CAD build for the part. Positions are in the model's coordinates, mm. Face numbers are marked on the shaded views. A direction names the side the tool comes from. Round coordinates to 2 decimals unless told otherwise and drop trailing zeros. Order: outer loops, then holes, each group sorted by start corner. A loop starts at its lowest first (then second) coordinate and runs counter-clockwise, first axis right, second up. Notation, with made-up numbers: (50, 20) -> (64, 20) arc R22 cw to (64, 26) -> close; hole circle Ø8 at (-12.5, -38). An arc over 180 degrees is marked (long way). Answer as CSV lines item,"result". Start each with the question number.
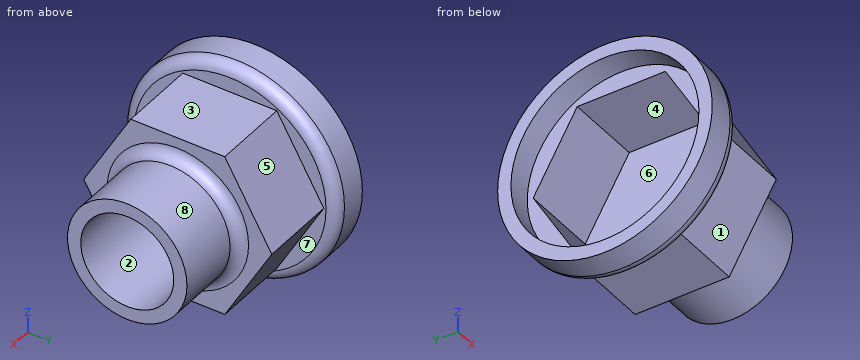
from build123d import *

# Parameters (mm, degrees)
F3_DEPTH = 7
F4_R     = 10.135693
F5_DEPTH = 13.801
F6_R     = 1
F7_R     = 1
F8_R     = 4.2
F9_DEPTH = 0.2


with BuildPart() as f1:
    # F0 (on Top) → F1 (revolve)
    with BuildSketch(Plane.XY):
        Polygon((0, 8.5), (0, 6.7), (7, 6.7), (7, 4.2), (15, 4.2), (15, 5.4), (8.2, 5.4), (8.2, 8.5), (1.2, 8.5), (1.2, 9.7), (-2.2, 9.7), (-2.2, 8.5), align=None)
    revolve(axis=Axis((9.6, 0, 0), (-1, 0, 0)))

    # F2 (on face) → F3 (cut)
    with BuildSketch(Plane(origin=(0, 0, 0), x_dir=(0, -1, 0), z_dir=(-1, 0, 0))):
        Polygon((3.983717, 6.9), (-3.983717, 6.9), (-7.967434, 0), (-3.983717, -6.9), (3.983717, -6.9), (7.967434, 0), align=None)
    extrude(amount=-F3_DEPTH, mode=Mode.SUBTRACT)

    # F4 (on face) → F5 (cut, through all)
    with BuildSketch(Plane.YZ.offset(1.2)):
        Circle(F4_R)
        Polygon((-8.5, 0), (-4.25, 7.361216), (4.25, 7.361216), (8.5, 0), (4.25, -7.361216), (-4.25, -7.361216), align=None, mode=Mode.SUBTRACT)
    extrude(amount=F5_DEPTH, mode=Mode.SUBTRACT)

    # F6
    f6_edges = [f1.edges().sort_by_distance(p)[0] for p in [
        (8.2, -5.4, 0),
    ]]
    fillet(f6_edges, radius=F6_R)

    # F7
    f7_edges = [f1.edges().sort_by_distance(p)[0] for p in [
        (1.2, -9.7, 0),
    ]]
    fillet(f7_edges, radius=F7_R)

    # F8 (on face) → F9 (join)
    with BuildSketch(Plane(origin=(7, 0, 0), x_dir=(0, -1, 0), z_dir=(-1, 0, 0))):
        Circle(F8_R)
    extrude(amount=-F9_DEPTH)


solid = f1.part
Item 1: Band-saw the part on D-D, the plane x = 0.75. Give the cut face in (y, z), and give its area (3 significant figures).
Item 2: Probe line 1 (Y direction, x = 11.25, z = 0); line 2 (Z direction, x = 3, y = -3.5); line 3 (Y direction, x = -1.35, z = 0). List the from-to ranges inside material, lowest first.
Item 3: Tool access for the marked faces 1, 2, 3, 4 and 5: list every direction of +Z, -Z, +X, -X, +Y, -Y with a clear straight run to the whole face (end or side of a thin tool).
Item 4: Mould opens along Z. For the marked faces 6, 7 and 8 say: released by +Z, released by -Z, zero draft, split by the parting line, or undercut.
Item 5: Band-saw the part on B-B, the plane y = 0. Give the cut face in (x, z).
Item 6: Pin check, flat tips, straight feed: pin 1 (2 mm diameter, centred on x = 5.5, y = 1.5, fed in from -Z); pin 2 (5 mm diameter, centred on x = 11, z = 4.5, fed in from +Y); pin 3 (2 mm diameter, centred on x = 2.5, y = 1, fed in from +Z). Stop position of each tip, or through.
Item 7: Band-saw the part on C-C, the plane x = 10.5. Give the cut face in (y, z).
Item 8: Band-saw the part on A-A, the plane x = 2.5. Give the cut face in (y, z).
Values:
1,outline,"circle Ø19.07 at (0, 0); hole (-7.97, 0) -> (-3.98, -6.9) -> (3.98, -6.9) -> (7.97, 0) -> (3.98, 6.9) -> (-3.98, 6.9) -> close"
1,area,"121 mm²"
2,line 1,"-5.4 to -4.2, 4.2 to 5.4"
2,line 2,"-7.36 to -6.9, 6.9 to 7.36"
2,line 3,"-9.7 to -8.5, 8.5 to 9.7"
3,face 1,"-Z, +X, -Y"
3,face 2,"+X"
3,face 3,"+Z, +X, +Y, -Y"
3,face 4,"-X"
3,face 5,"+Z, +X, +Y"
4,face 6,"undercut"
4,face 7,"zero draft"
4,face 8,"split by the parting line"
5,outline,"(-2.2, -9.7) -> (0.2, -9.7) arc R1 ccw to (1.2, -8.7) -> (1.2, -7.36) -> (8.2, -7.36) -> (8.2, -6.4) arc R1 cw to (9.2, -5.4) -> (15, -5.4) -> (15, -4.2) -> (7.2, -4.2) -> (7.2, 4.2) -> (15, 4.2) -> (15, 5.4) -> (9.2, 5.4) arc R1 cw to (8.2, 6.4) -> (8.2, 7.36) -> (1.2, 7.36) -> (1.2, 8.7) arc R1 ccw to (0.2, 9.7) -> (-2.2, 9.7) -> (-2.2, 8.5) -> (0, 8.5) -> (0, 6.9) -> (7, 6.9) -> (7, -6.9) -> (0, -6.9) -> (0, -8.5) -> (-2.2, -8.5) -> close"
6,pin 1,"z = -7.36"
6,pin 2,"y = 5.02"
6,pin 3,"z = 7.36"
7,outline,"circle Ø10.8 at (0, 0); hole circle Ø8.4 at (0, 0)"
8,outline,"(-8.5, 0) -> (-4.25, -7.36) -> (4.25, -7.36) -> (8.5, 0) -> (4.25, 7.36) -> (-4.25, 7.36) -> close; hole (-7.97, 0) -> (-3.98, -6.9) -> (3.98, -6.9) -> (7.97, 0) -> (3.98, 6.9) -> (-3.98, 6.9) -> close"
